Work out the finished part from the listing and answer in its coordinate system (mm). A direction names the side the tool comes from. Coordinates: 2 decimals unless noted, no trailing zeros. Order: outer loops, then holes, each group sorted by start corner. A loop starts at its lowest first (then second) coordinate and runs counter-clockwise, first axis right, second up. Notation, with made-up numbers: (58.25, 32.25) - (80.25, 32.25) arc R31 cw to (80.25, 63.25) - close; hole circle Ø8 at (48, 12). An arc over 180 degrees is marked (long way). Use CSV: the item, a comma, the result in double quotes. Start each with the question number.
from build123d import *

# Parameters (mm, degrees)
SKETCH1_R           = 74
BOSS_EXTRUDE1_DEPTH = 30
SKETCH2_R           = 10
CUT_EXTRUDE1_DEPTH  = 80
SKETCH3_R           = 10
CUT_EXTRUDE2_DEPTH  = 80
SKETCH6_R           = 3
CUT_EXTRUDE4_DEPTH  = 30
SCALE1_SCALE        = 0.75


with BuildPart() as part:
    # Sketch1 → Boss-Extrude1 (new body)
    with BuildSketch(Plane(origin=(0, 0, 0), x_dir=(1, 0, 0), z_dir=(0, 1, 0))):
        Circle(SKETCH1_R)
    extrude(amount=BOSS_EXTRUDE1_DEPTH)

    # Sketch2 → Cut-Extrude1 (cut)
    with BuildSketch(Plane(origin=(0, 0, 0), x_dir=(0, 0, -1), z_dir=(1, 0, 0))):
        with Locations((45, 15)):
            Circle(SKETCH2_R)
    extrude(amount=-CUT_EXTRUDE1_DEPTH, mode=Mode.SUBTRACT)

    # Sketch3 → Cut-Extrude2 (cut)
    with BuildSketch(Plane(origin=(0, 0, 0), x_dir=(0, 0, -1), z_dir=(1, 0, 0))):
        with Locations((-45, 15)):
            Circle(SKETCH3_R)
    extrude(amount=CUT_EXTRUDE2_DEPTH, mode=Mode.SUBTRACT)

    # Sketch6 → Cut-Extrude4 (cut)
    with BuildSketch(Plane(origin=(0, 30, 0), x_dir=(1, 0, 0), z_dir=(0, 1, 0))):
        Circle(SKETCH6_R)
    extrude(amount=-CUT_EXTRUDE4_DEPTH, mode=Mode.SUBTRACT)


with BuildPart() as part_1:
    # Scale1: scaled about (-3.1666e-05, 14.999981435, 5.427e-06)
    add(part.part.scale(SCALE1_SCALE).moved(Location((-7.916e-06, 3.749995359, 1.357e-06))))


solid = part_1.part
1) For a pull along X with two mould halves and no side action, classify faces 1 (the face through (2.146, 15.157, -0.676)), 2 (the face through (25.61, 14.84, 49.24)), 3 (the face through (24.108, 17.253, 26.596)) as +X half, -X half, draft (parallel to the pull), parting line (faces both ways), or undercut.
2) The part is cut by section B-B on x = 16. Determine the outline of the cut face in (y, z).
3) The part is cut by section D-D on z = 19.5. Determine the outline of the cut face in (x, y).
4) For faces 4 (the face through (0, 15, -34)), 5 (the face through (0, 15, 34)), 6 (the face through (-1, 26.25, 12)), determine the directions among +Z, -Z, +X, -X, +Y, -Y from which every point of the face is accessible in a straight line to the end or side of a thin tool.
5) The part is cut by section C-C on x = 41.5. Determine the outline of the cut face in (y, z).
6) The part is cut by section A-A on y = 13.5. Determine the outline of the cut face in (x, z).
7) Flat-ended cylindrical pins translate along their axes: P1, Ø2.5, axis at x = 0, z = 0, coming from the +Y side; P2, Ø12, axis at y = 15, z = -33.75, coming from the -X side; P3, Ø12, axis at x = -13.5, y = 10.5, coming from the -Z side; P4, Ø1.5, axis at y = 15, z = -13, coming from the +X side. Find the tip coordinate at first contact, or state that the pin passes through.
8) Straight lines are drawn through the part: line 1 (Y direction, x = -22, z = -31.5); line 2 (Z direction, x = 9, y = 16); line 3 (Z direction, x = 26, y = 8.25). For each, find the intervals that lie inside material, in ascending order. Write a range as [from, to].
Answer key:
1,face 1,"undercut"
1,face 2,"parting line"
1,face 3,"draft"
2,outline,"(3.75, -53.14) - (26.25, -53.14) - (26.25, 53.14) - (3.75, 53.14) - close; hole circle Ø15 at (15, 33.75)"
3,outline,"(-51.96, 3.75) - (51.96, 3.75) - (51.96, 26.25) - (-51.96, 26.25) - close"
4,face 4,"-X"
4,face 5,"+X"
4,face 6,"+Z, -Z, +X, -X, +Y"
5,outline,"(3.75, -36.85) - (26.25, -36.85) - (26.25, 36.85) - (21.83, 36.85) arc R7.5 cw (long way) to (8.17, 36.85) - (3.75, 36.85) - close"
6,outline,"(-48.82, -26.4) - (0, -26.4) - (0, -41.1) - (-37.3, -41.1) arc R55.5 ccw to (48.82, 26.4) - (0, 26.4) - (0, 41.1) - (37.3, 41.1) arc R55.5 ccw to start; hole circle Ø4.5 at (0, 0)"
7,P1,"through"
7,P2,"x = 0"
7,P3,"z = -54.99"
7,P4,"x = 54.13"
8,line 1,"[3.75, 7.85], [22.15, 26.25]"
8,line 2,"[-54.77, 26.32], [41.18, 54.77]"
8,line 3,"[-49.03, 30.48], [37.02, 49.03]"
